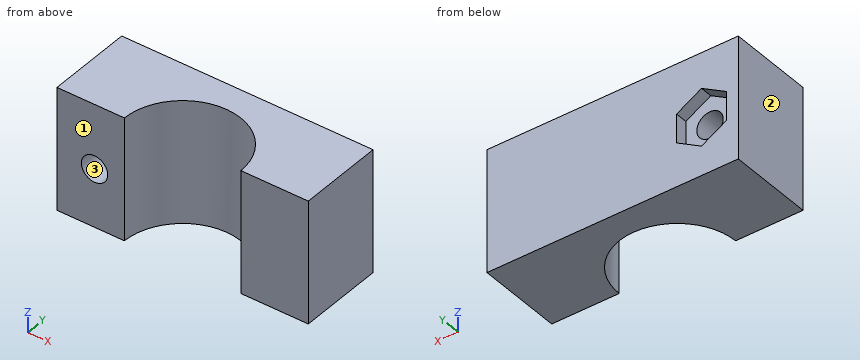
Autodesk Inventor part; units mm, degrees
ref_plane "YZ Plane" through (0, 0, 0) normal (1, 0, 0) x (0, 1, 0)
ref_plane "XZ Plane" through (0, 0, 0) normal (0, 1, 0) x (-1, 0, 0)
ref_plane "XY Plane" through (0, 0, 0) normal (0, 0, 1) x (1, 0, 0)
sketch "Sketch1" plane through (0, 0, 0) normal (0, 1, 0) x (-1, 0, 0)
  line L0 (0, 0) -> (-20.51, 0)
  line L1 (-20.51, 0) -> (-20.51, -10)
  line L2 (-20.51, -10) -> (0, -10)
  line L3 (0, -10) -> (0, 0)
  dimension "d0" = 20.51
  dimension "d1" = 10
extrude "Extrusion1" add sketch "Sketch1" along normal blind 7
sketch "Sketch2" plane through (0, 0, 0) normal (0, 0, 1) x (1, 0, 0)
  line L0 (20.51, 0) -> (0, 0)
  circle A0 centre (10.255, 0) radius 4.75
  dimension "d4" = 9.5
extrude "Extrusion2" cut sketch "Sketch2" against normal through all
sketch "Sketch3" plane through (0, 7, 0) normal (0, 1, 0) x (1, 0, 0)
  line L0 (3, 7.6072) -> (5.0352, 6.4322)
  line L1 (5.0352, 6.4322) -> (5.0352, 4.0822)
  line L2 (5.0352, 4.0822) -> (3, 2.9072)
  line L3 (3, 2.9072) -> (0.9648, 4.0822)
  line L4 (0.9648, 4.0822) -> (0.9648, 6.4322)
  line L5 (0.9648, 6.4322) -> (3, 7.6072)
  point P0 (0, 0)
  point P1 (3, 5.2572)
extrude "Extrusion3" cut sketch "Sketch3" against normal blind 1
sketch "Sketch4" plane through (0, 6, 0) normal (0, 1, 0) x (1, 0, 0)
  circle A0 centre (3.0647, 5.2572) radius 1.075
  point P0 (0, 0)
  dimension "d10" = 2.15
extrude "Extrusion4" cut sketch "Sketch4" against normal through all
properties part number "dg_clampv2"
CAD build for the part. Positions are in the model's coordinates, mm. Face numbers are marked on the shaded views. Round coordinates to 2 decimals unless told otherwise and drop trailing zeros. Order: outer loops, then holes, each group sorted by start corner. A loop starts at its lowest first (then second) coordinate and runs counter-clockwise, first axis right, second up. Notation, with made-up numbers: (28.25, -21.75) - (77.25, -21.75) arc R21 ccw to (77.25, -15.75) - close; hole circle Ø9 at (5.5, 15). An arc over 180 degrees is marked (long way). Answer as CSV lines item,"result". Start each with the question number.
1. Drill centre lines: L1, parallel to X at y = 3.25, z = -4.75; L2, parallel to X at y = 2.75, z = -1.5; L3, parallel to X at y = 3, z = -7. Where is each one in solid material? Low to high. Write a range as [from, to].
2. Saw through at A-A, the plane y = 0.5. Write the cut outline in (x, z) (3 decimals), and give its area (3 significant figures).
3. Saw through at B-B, the plane z = -6. Write the cut outline in (x, y) (3 decimals), and give its area (3 significant figures).
4. Pin check, flat tip, straight feed: pin 1 (2.5 mm diameter, centred on x = 3.06, z = -5.26, fed in from +Y). Stop position of the tip, or through.
5. Saw through at C-C, the plane z = -2. Write the cut outline in (x, y) (3 decimals).
6. Pull direction X, two halves, no side cores. Call the marked faces 1, 2 and 3: +X half, -X half, draft (parallel to the pull), parting line (faces both ways), or undercut.
7. Saw through at D-D, the plane y = 3. Write the cut outline in (x, z) (3 decimals), and give its area (3 significant figures).
Model answer:
1,L1,"x = [0, 2.12], [4.01, 6.79], [13.72, 20.51]"
1,L2,"x = [0, 6.38], [14.13, 20.51]"
1,L3,"x = [0, 6.57], [13.94, 20.51]"
2,outline,"(0, -10) - (5.531, -10) - (5.531, 0) - (0, 0) - close; (14.979, -10) - (20.51, -10) - (20.51, 0) - (14.979, 0) - close; hole circle Ø2.15 at (3.065, -5.257)"
2,area,"107 mm²"
3,outline,"(0, 0) - (2.288, 0) - (2.288, 6) - (0.965, 6) - (0.965, 7) - (0, 7) - close; (3.842, 0) - (5.505, 0) arc R4.75 cw to (15.005, 0) - (20.51, 0) - (20.51, 7) - (5.035, 7) - (5.035, 6) - (3.842, 6) - close"
3,area,"94.7 mm²"
4,pin 1,"stops at y = 6"
5,outline,"(0, 0) - (5.505, 0) arc R4.75 cw to (15.005, 0) - (20.51, 0) - (20.51, 7) - (0, 7) - close"
6,face 1,"draft"
6,face 2,"-X half"
6,face 3,"undercut"
7,outline,"(0, -10) - (6.572, -10) - (6.572, 0) - (0, 0) - close; (13.938, -10) - (20.51, -10) - (20.51, 0) - (13.938, 0) - close; hole circle Ø2.15 at (3.065, -5.257)"
7,area,"128 mm²"
